Here's how the part is built. I have some questions about the finished solid (model axes, mm). Face numbers are marked on the shaded views. A direction names the side the tool comes from. Round coordinates to 2 decimals unless told otherwise and drop trailing zeros. Order: outer loops, then holes, each group sorted by start corner. A loop starts at its lowest first (then second) coordinate and runs counter-clockwise, first axis right, second up. Notation, with made-up numbers: M 15,-16 L 32,-16 A24 cw 32,-3 Z; hole C 74,33 d11. An arc over 180 degrees is marked long. Answer as CSV lines item,"result". Start each with the question number.
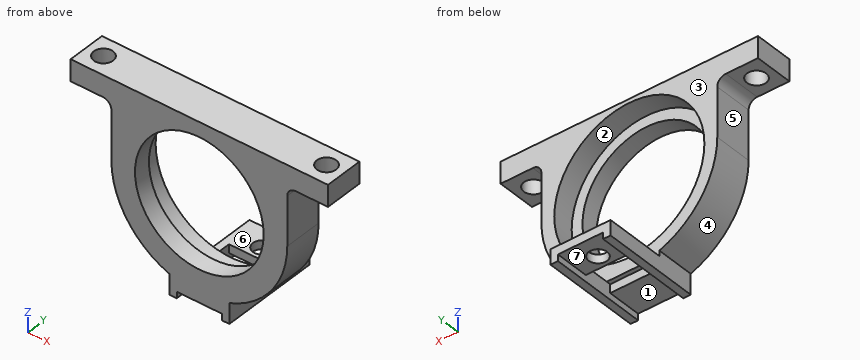
```python
from build123d import *

# Parameters (mm, degrees)
SKETCH1_R                 = 17.5
BOSS_EXTRUDE1_DEPTH       = 5
SKETCH3_R                 = 15
BOSS_EXTRUDE2_DEPTH       = 4
FILLET2_R                 = 2
F_8_CLEARANCE_HOLE1_D     = 4.4958
F_8_CLEARANCE_HOLE1_DEPTH = 23.75
F_8_CLEARANCE_HOLE1_TIP   = 1.350674586
BOSS_EXTRUDE3_DEPTH       = 9
BOSS_EXTRUDE4_DEPTH       = 14
SKETCH8_R                 = 2.1463
CUT_EXTRUDE1_DEPTH        = 41.9
SKETCH9_W                 = 10.52
SKETCH9_H                 = 7
CUT_EXTRUDE2_DEPTH        = 2


with BuildPart() as part:
    # Sketch1 → Boss-Extrude1 (new body)
    with BuildSketch(Plane(origin=(0, 0, 0), x_dir=(1, 0, 0), z_dir=(0, 1, 0))):
        with BuildLine():
            ThreePointArc((-20.5, 18.4), (0, 38.9), (20.5, 18.4))
            Line((20.5, 18.4), (20.5, 5))
            Line((20.5, 5), (30, 5))
            Line((30, 5), (30, 0))
            Line((30, 0), (0, 0))
            Line((0, 0), (-30, 0))
            Line((-30, 0), (-30, 5))
            Line((-30, 5), (-20.5, 5))
            Line((-20.5, 5), (-20.5, 18.4))
        make_face()
        with Locations((0, 18.4)):
            Circle(SKETCH1_R, mode=Mode.SUBTRACT)
    extrude(amount=BOSS_EXTRUDE1_DEPTH)

    # Sketch3 → Boss-Extrude2 (add)
    with BuildSketch(Plane.XZ):
        with BuildLine():
            Line((20.5, -18.4), (20.5, -5))
            Line((20.5, -5), (30, -5))
            Line((30, -5), (30, 0))
            Line((30, 0), (-30, 0))
            Line((-30, 0), (-30, -5))
            Line((-30, -5), (-20.5, -5))
            Line((-20.5, -5), (-20.5, -18.4))
            ThreePointArc((-20.5, -18.4), (0, -38.9), (20.5, -18.4))
        make_face()
        with Locations((0, -18.4)):
            Circle(SKETCH3_R, mode=Mode.SUBTRACT)
    extrude(amount=BOSS_EXTRUDE2_DEPTH)

    # Fillet2
    fillet2_edges = [part.edges().sort_by_distance(p)[0] for p in [
        (20.5, 0.5, -5),
        (-20.5, 0.5, -5),
    ]]
    fillet(fillet2_edges, radius=FILLET2_R)

    # #8 Clearance Hole1
    with Locations(Plane(origin=(0, 0, -5), x_dir=(-1, 0, 0), z_dir=(0, 0, -1))):
        with Locations((-26, 0.5), (26, 0.5)):
            Hole(F_8_CLEARANCE_HOLE1_D / 2, depth=F_8_CLEARANCE_HOLE1_DEPTH)
            with Locations((0, 0, -(F_8_CLEARANCE_HOLE1_DEPTH + F_8_CLEARANCE_HOLE1_TIP / 2))):  # 118° drill point
                Cone(0, F_8_CLEARANCE_HOLE1_D / 2, F_8_CLEARANCE_HOLE1_TIP, mode=Mode.SUBTRACT)

    # Sketch6 → Boss-Extrude3 (add)
    with BuildSketch(Plane.XZ.offset(4)):
        with BuildLine():
            Line((7, -37.667848868), (7, -42.4))
            Line((7, -42.4), (5.26, -42.4))
            Line((5.26, -42.4), (5.26, -40.9))
            Line((5.26, -40.9), (-5.26, -40.9))
            Line((-5.26, -40.9), (-5.26, -42.4))
            Line((-5.26, -42.4), (-7, -42.4))
            Line((-7, -42.4), (-7, -37.667848868))
            ThreePointArc((-7, -37.667848868), (0, -38.9), (7, -37.667848868))
        make_face()
    extrude(amount=-BOSS_EXTRUDE3_DEPTH)

    # Sketch7 → Boss-Extrude4 (add)
    with BuildSketch(Plane(origin=(0, 5, 0), x_dir=(1, 0, 0), z_dir=(0, 1, 0))):
        Polygon((5.26, 42.4), (7, 42.4), (7, 38.9), (-7, 38.9), (-7, 42.4), (-5.26, 42.4), (-5.26, 40.9), (5.26, 40.9), align=None)
    extrude(amount=BOSS_EXTRUDE4_DEPTH)

    # Sketch8 → Cut-Extrude1 (cut, through all)
    with BuildSketch(Plane(origin=(0, 0, -40.9), x_dir=(-1, 0, 0), z_dir=(0, 0, -1))):
        with Locations((0, 14)):
            Circle(SKETCH8_R)
    extrude(amount=-CUT_EXTRUDE1_DEPTH, mode=Mode.SUBTRACT)

    # Sketch9 → Cut-Extrude2 (cut)
    with BuildSketch(Plane(origin=(0, 0, -40.9), x_dir=(-1, 0, 0), z_dir=(0, 0, -1))):
        with Locations((0, 7.5)):
            Rectangle(SKETCH9_W, SKETCH9_H)
    extrude(amount=-CUT_EXTRUDE2_DEPTH, mode=Mode.SUBTRACT)


solid = part.part
```
Item 1: For P1, Ø8, axis at y = 9.5, z = -33, coming from the +X side; P2, Ø5, axis at x = 11.5, y = -1, coming from the -Z side; P3, Ø6, axis at x = 26, y = 0.5, coming from the +Z side; P4, Ø1.5, axis at x = 12, y = 4.5, coming from the -Z side, each with a flat end and sliding along its axis, tell me the tip position at first contact or that it passes through.
Item 2: We'd pull the mould along X, two halves only. Please class the marked faces 1, 2, 3 and 4: pulls with the +X half, pulls with the -X half, needs draft (parallel to the pull), parting line crosses it, or undercut.
Item 3: If we section it at C-C on y = 14: Please give me the cut outline in (x, z), and give its area (3 significant figures).
Item 4: If we section it at D-D on z = -17: Please give me the cut outline in (x, y), and give its area (3 significant figures).
Item 5: If I drill on line 1 along Z through (x, y) = (0, -2.4); line 2 along Y through (x, z) = (16.5, -20.5); line 3 along Y through (x, z) = (26, -2), over which ranges is the centre line in solid material (lowest first)?
Item 6: If we section it at A-A on x = 26: Please give me the cut outline in (y, z), and give its area (3 significant figures).
Item 7: Which directions (+Z, -Z, +X, -X, +Y, -Y) give clear straight access to the entire face, cutting with the end or side of a thin tool? Please do the marked faces 5, 6 and 7.
Item 8: If we section it at B-B on x = 0: Please give me the cut outline in (y, z), and give its area (3 significant figures).
Geometry says:
1,P1,"through"
1,P2,"z = -36.82"
1,P3,"z = 0"
1,P4,"z = -35.54"
2,face 1,"undercut"
2,face 2,"undercut"
2,face 3,"needs draft"
2,face 4,"pulls with the -X half"
3,outline,"M -7,-42.4 L -5.26,-42.4 L -5.26,-40.9 L -2.15,-40.9 L -2.15,-38.9 L -7,-38.9 Z; M 2.15,-40.9 L 5.26,-40.9 L 5.26,-42.4 L 7,-42.4 L 7,-38.9 L 2.15,-38.9 Z"
3,area,"24.6 mm²"
4,outline,"M -20.5,-4 L -14.93,-4 L -14.93,0 L -17.44,0 L -17.44,5 L -20.5,5 Z; M 14.93,-4 L 20.5,-4 L 20.5,5 L 17.44,5 L 17.44,0 L 14.93,0 Z"
4,area,"75.1 mm²"
5,line 1,"-40.9 to -33.4, -3.4 to 0"
5,line 2,"-4 to 0"
5,line 3,"-4 to -1.75, 2.75 to 5"
6,outline,"M -4,-5 L -1.75,-5 L -1.75,0 L -4,0 Z; M 2.75,-5 L 5,-5 L 5,0 L 2.75,0 Z"
6,area,"22.5 mm²"
7,face 5,"-Z, -X, +Y, -Y"
7,face 6,"+Z, +X, -X, +Y"
7,face 7,"-Z, +Y, -Y"
8,outline,"M -4,-40.9 L 4,-40.9 L 4,-38.9 L 5,-38.9 L 5,-35.9 L 0,-35.9 L 0,-33.4 L -4,-33.4 Z; M -4,-3.4 L 0,-3.4 L 0,-0.9 L 5,-0.9 L 5,0 L -4,0 Z; M 11,-40.9 L 11.85,-40.9 L 11.85,-38.9 L 11,-38.9 Z; M 16.15,-40.9 L 19,-40.9 L 19,-38.9 L 16.15,-38.9 Z"
8,area,"78.5 mm²"
